Can you work these out from the model? Positions are in its coordinate system, mm. Give positions to 0.01 mm unless a question says otherwise; leave off trailing zeros. Order: outer loops, then holes, each group sorted by start corner. A loop starts at its lowest first (then second) coordinate and runs counter-clockwise, first axis right, second up. Notation, with made-up numbers: (-27.5, 77.25) - (8.5, 77.25) arc R23 ccw to (8.5, 110.25) - close; hole circle Ø8 at (-33.5, 28). An arc over 180 degrees is marked (long way). Return JSON: item names as keys, results as strings.
```python
from build123d import *

# Parameters (mm, degrees)
PAD012_DEPTH            = 3
SKETCH090_R             = 27.75
POCKET039_DEPTH         = 0.001
POCKET039_DEPTH_BACK    = 3.001
POCKET040_DEPTH         = 0.001
POCKET040_DEPTH_BACK    = 3.001
BODY081_PLACEMENT_ANGLE = 90


with BuildPart() as part:
    # Sketch089 → Pad012 (new body)
    with BuildSketch(Plane.XY):
        with BuildLine():
            ThreePointArc((-184, -130), (-182.535534, -133.535534), (-179, -135))
            Line((179, -135), (-179, -135))
            ThreePointArc((179, -135), (182.535534, -133.535534), (184, -130))
            Line((184, 130), (184, -130))
            ThreePointArc((184, 130), (182.535534, 133.535534), (179, 135))
            Line((-179, 135), (179, 135))
            ThreePointArc((-179, 135), (-182.535534, 133.535534), (-184, 130))
            Line((-184, -130), (-184, 130))
        make_face()
    extrude(amount=PAD012_DEPTH)

    # Sketch090 → Pocket039 (cut, two sides)
    with BuildSketch(Plane(origin=(-140, 90, 0), x_dir=(1, 0, 0), z_dir=(0, 0, 1))) as pocket039_sk:
        Circle(SKETCH090_R)
    extrude(amount=-POCKET039_DEPTH, mode=Mode.SUBTRACT)
    extrude(pocket039_sk.sketch, amount=POCKET039_DEPTH_BACK, mode=Mode.SUBTRACT)

    # Sketch091 → Pocket040 (cut, two sides)
    with BuildSketch(Plane.XY) as pocket040_sk:
        with BuildLine():
            Line((184, 135), (149, 135))
            ThreePointArc((154, 130), (152.535534, 133.535534), (149, 135))
            Line((154, 130), (154, 70))
            ThreePointArc((154, 70), (155.464466, 66.464466), (159, 65))
            Line((159, 65), (179, 65))
            ThreePointArc((184, 60), (182.535534, 63.535534), (179, 65))
            Line((184, 60), (184, 135))
        make_face()
    extrude(amount=-POCKET040_DEPTH, mode=Mode.SUBTRACT)
    extrude(pocket040_sk.sketch, amount=POCKET040_DEPTH_BACK, mode=Mode.SUBTRACT)


with BuildPart() as part_1:
    # Body081 placement: moved
    add(part.part.moved(Location((1341, 1390, 0))).rotate(Axis((1341, 1390, 0), (0, 0, 1)), BODY081_PLACEMENT_ANGLE))


solid = part_1.part
```
1. Thinking about a two-plate mould opening in X: for faces 1 (the face through (1223.486, 1246.388, 1.479)), 2 (the face through (1339, 1387, 3)), which applies, +X half, -X half, draft (parallel to the pull), parting line (faces both ways), or undercut?
Checks:
{"face 1": "undercut", "face 2": "draft"}
2. Suppose I cut it at C-C (z = 2.2). List the corners of the cut face in (x, y) for me, plus the area to 3 significant figures.
Checks:
{"outline": "(1206, 1211) arc R5 ccw to (1211, 1206) - (1471, 1206) arc R5 ccw to (1476, 1211) - (1476, 1569) arc R5 ccw to (1471, 1574) - (1281, 1574) arc R5 ccw to (1276, 1569) - (1276, 1549) arc R5 cw to (1271, 1544) - (1211, 1544) arc R5 ccw to (1206, 1539) - close; hole circle Ø55.5 at (1251, 1250)", "area": "94,800 mm^2"}
3. Suppose I cut it at B-B (x = 1251). List the corners of the cut face in (y, z) for me.
Checks:
{"outline": "(1206, 0) - (1222.25, 0) - (1222.25, 3) - (1206, 3) - close; (1277.75, 0) - (1544, 0) - (1544, 3) - (1277.75, 3) - close"}
4. If I drill on L1, parallel to X at y = 1250, z = 1.8; L2, parallel to X at y = 1551.5, z = 1.6; L3, parallel to Y at x = 1242.5, z = 0.8, over which ranges is the centre line in solid material (lowest first)? Write a range as [from, to].
Checks:
{"L1": "[1206, 1223.25], [1278.75, 1476]", "L2": "[1276, 1476]", "L3": "[1206, 1223.58], [1276.42, 1544]"}
5. For pin 1 Ø10 at (x, y) = (1337.5, 1298.5) entering from -Z; pin 2 Ø0.9 at (y, z) = (1563, 2) entering from -X, each with a flat end and sliding along its axis, tell me the tip position at first contact or that it passes through.
Checks:
{"pin 1": "z = 0", "pin 2": "x = 1276"}
6. Suppose I cut it at A-A (y = 1250). List the corners of the cut face in (x, z) for me.
Checks:
{"outline": "(1206, 0) - (1223.25, 0) - (1223.25, 3) - (1206, 3) - close; (1278.75, 0) - (1476, 0) - (1476, 3) - (1278.75, 3) - close"}
